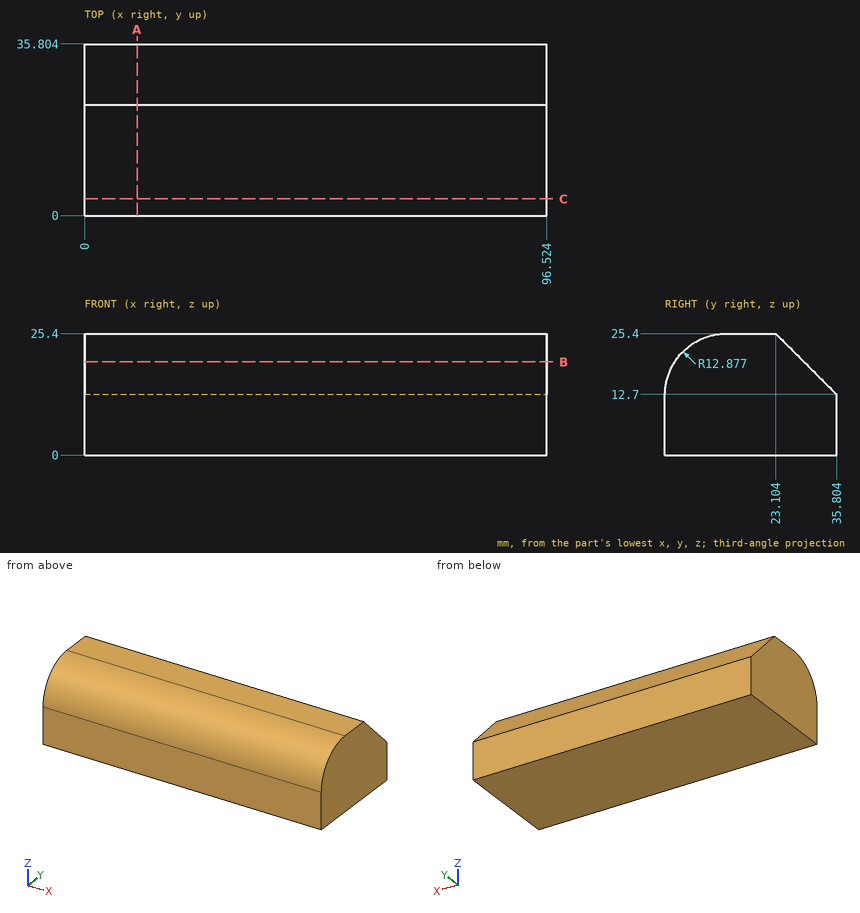
The drawing under review shows one solid part. Ordinate dimensions are in mm from its lowest x, y, z. Coordinates: 2 decimals unless noted, no trailing zeros. Order: outer loops, then holes, each group sorted by start corner. A loop starts at its lowest first (then second) coordinate and runs counter-clockwise, first axis right, second up. Notation, with made-up numbers: (30.5, 80) - (70.5, 80) arc R17 ccw to (70.5, 99) - close; hole circle Ø11 at (-1, -12). An arc over 180 degrees is marked (long way). Put each result on its own line as item: value.
1) Take a section at B-B, the plane z = 19.5. Give the boundary of the cut face in (x, y), and give its area (3 significant figures).
Response values:
outline: (0, 2.05) - (96.52, 2.05) - (96.52, 29) - (0, 29) - close
area: 2,600 mm²
2) Insertion check: P1, Ø12, axis at y = 7, z = 16, coming from the -X side. The pin has a flat end and moves straight along its axis. Give the tip position at first contact, or say it passes through.
Response values:
P1: stops at x = 0
3) Wall thickness on L1, parallel to Z at x = 30.5, y = 29 (1 decimal); L2, parallel to Z at x = 33, y = 7; L3, parallel to Y at x = 56, z = 17.5 (1 decimal): over which ranges is each line inside the solid? List them lowest first. Write a range as from..to.
Response values:
L1: z = 0..19.5
L2: z = 0..23.98
L3: y = 1..31
4) Take a section at C-C, the plane y = 3.5. Give the boundary of the cut face in (x, z), and give its area (3 significant figures).
Response values:
outline: (0, 0) - (96.52, 0) - (96.52, 21.35) - (0, 21.35) - close
area: 2,060 mm²
5) Take a section at A-A, the plane x = 11. Give the boundary of the cut face in (y, z) (1 decimal), and give its area (3 significant figures).
Response values:
outline: (0, 0) - (35.8, 0) - (35.8, 12.7) - (23.1, 25.4) - (12.9, 25.4) arc R12.9 ccw to (0, 12.5) - close
area: 793 mm²
